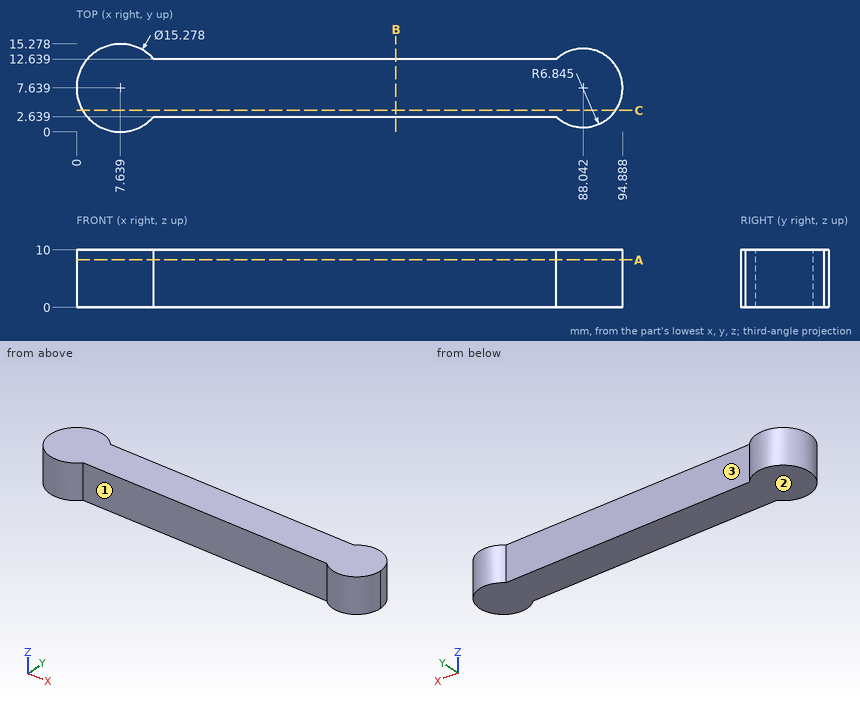
Check sheet for the drawn part. Datum: minimum x, y, z corner. Units: mm. Give positions to 0.01 mm unless a question says otherwise; leave off trailing zeros. Write each loop counter-clockwise with the first axis right and the second up, starting at its lowest first coordinate (ties: lowest second). Pieces come first, ordered by that corner, then holes. Notation, with made-up numbers: (-31.75, -26.75) -> (2.25, -26.75) arc R22 cw to (2.25, -11.75) -> close; hole circle Ø3 at (58, 59). An arc over 180 degrees is marked (long way). Use one line per item in the form item = value. Start each with the question number.
1. Mould release check, pull along X, two halves, no side actions. Record for the marked faces 1, 2 and 3: pulls with the +X half, pulls with the -X half, needs draft (parallel to the pull), parting line crosses it, or undercut.
2. Section check B-B (x = 55.5). Record the cut outline in (y, z), and give its area (3 significant figures).
3. Section check C-C (y = 3.75). Record the cut outline in (x, z) (1 decimal).
4. Section check A-A (z = 8.25). Record the cut outline in (x, y) (1 decimal).
5. Go/stop test with flat-tipped pins: P1, Ø6, axis at x = 54.5, z = 6, coming from the +Y side; P2, Ø3, axis at y = 2.5, z = 5, coming from the +X side; P3, Ø1.5, axis at x = 44, z = 4, coming from the -Y side. Record where each tip stops, or that it passes through.
6. Thickness scan on line 1 along Y through (x, z) = (14, 3); line 2 along Y through (x, z) = (88, 1.75) (1 decimal); line 3 along X through (y, z) = (8, 2.75). Record the ranges inside material, lowest first. Write a range as from..to.
Conclusion:
q1.face_1 = undercut
q1.face_2 = needs draft
q1.face_3 = undercut
q2.outline = (2.64, 0) -> (12.64, 0) -> (12.64, 10) -> (2.64, 10) -> close
q2.area = 100 mm²
q3.outline = (1.1, 0) -> (93.7, 0) -> (93.7, 10) -> (1.1, 10) -> close
q4.outline = (13.4, 2.6) -> (83.4, 2.6) arc R6.8 ccw (long way) to (83.4, 12.6) -> (13.4, 12.6) arc R7.6 ccw (long way) to start
q5.P1 = 12.64
q5.P2 = 93.84
q5.P3 = 2.64
q6.line_1 = 2.64..12.64
q6.line_2 = 0.8..14.5
q6.line_3 = 0.01..94.88
